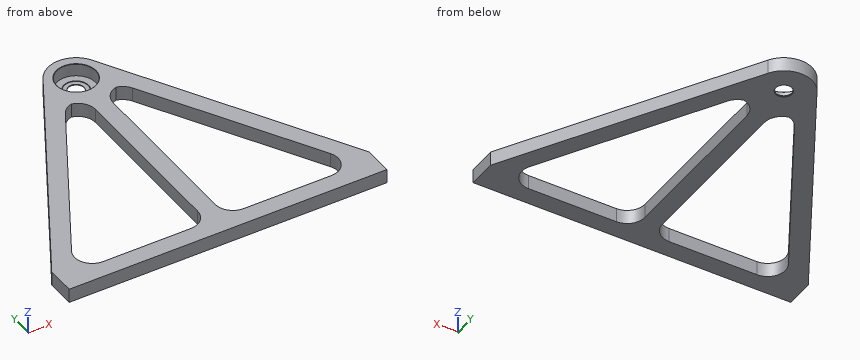
from build123d import *

# Parameters (mm, degrees)
BOSS_EXTRUDE1_DEPTH = 4
SKETCH2_R           = 11.05
CUT_EXTRUDE1_DEPTH  = 7.2
SKETCH3_R           = 7
CUT_EXTRUDE2_DEPTH  = 0.2
SKETCH4_R           = 4.5
CUT_EXTRUDE3_DEPTH  = 186.073210739
CHAMFER1_SIZE       = 0.2
CUT_EXTRUDE4_DEPTH  = 186.09817215
SKETCH8_W           = 10
SKETCH8_H           = 114
EXTRUDE_THIN1_DEPTH = 8
FILLET1_R           = 10
SKETCH6_OUTSIDE_W   = 251.144
SKETCH6_OUTSIDE_H   = 208.536
SKETCH6_OUTSIDE_W_2 = 180
SKETCH6_OUTSIDE_H_2 = 156
CUT_EXTRUDE5_DEPTH  = 186.09817215


# Some blends are built 0.0001 mm under size
with BuildPart() as part:
    # Sketch1 → Boss-Extrude1 (new, symmetric)
    with BuildSketch(Plane.XY):
        with BuildLine():
            Line((0, 0), (-99.304246301, 0))
            Line((-99.304246301, 0), (-13.856406461, 148))
            ThreePointArc((-13.856406461, 148), (0, 156), (13.856406461, 148))
            Line((13.856406461, 148), (99.304246301, 0))
            Line((99.304246301, 0), (0, 0))
        make_face()
    extrude(amount=BOSS_EXTRUDE1_DEPTH, both=True)

    # Sketch2 → Cut-Extrude1 (cut)
    with BuildSketch(Plane.XY.offset(4)):
        with Locations((0, 140)):
            Circle(SKETCH2_R)
    extrude(amount=-CUT_EXTRUDE1_DEPTH, mode=Mode.SUBTRACT)

    # Sketch3 → Cut-Extrude2 (cut)
    with BuildSketch(Plane.XY.offset(-3.2)):
        with Locations((0, 140)):
            Circle(SKETCH3_R)
    extrude(amount=-CUT_EXTRUDE2_DEPTH, mode=Mode.SUBTRACT)

    # Sketch4 → Cut-Extrude3 (cut, through all)
    with BuildSketch(Plane.XY.offset(-3.4)):
        with Locations((0, 140)):
            Circle(SKETCH4_R)
    extrude(amount=-CUT_EXTRUDE3_DEPTH, mode=Mode.SUBTRACT)

    # Chamfer1
    chamfer1_edges = [part.edges().sort_by_distance(p)[0] for p in [
        (-11.05, 140, 4),
        (-7, 140, -3.4),
        (-4.5, 140, -4),
    ]]
    chamfer(chamfer1_edges, length=CHAMFER1_SIZE - 0.0001)  # a hair under: the kernel refuses the full size

    # Sketch5 → Cut-Extrude4 (cut, through all)
    with BuildSketch(Plane.XY.offset(4)):
        Polygon((-16.165807537, 124), (16.165807537, 124), (81.983738225, 10), (-81.983738225, 10), align=None)
    extrude(amount=-CUT_EXTRUDE4_DEPTH, mode=Mode.SUBTRACT)

    # Sketch8 → Extrude-Thin1 (add)
    with BuildSketch(Plane.XY.offset(4)):
        with Locations((0, 67)):
            Rectangle(SKETCH8_W, SKETCH8_H)
    extrude(amount=-EXTRUDE_THIN1_DEPTH)

    # Fillet1
    # the kernel refuses this fillet: 10 mm, written as the material it adds along each edge
    with BuildSketch(Plane(origin=(81.983738225, 10, 4), x_dir=(-0.5000000000000037, 0.8660254037844365, 0), z_dir=(0, 0, -1)), Plane(origin=(-81.983738225, 10, 4), x_dir=(1, 0, 0), z_dir=(0, 0, -1))) as fillet1_piece_1:
        with BuildLine():
            CenterArc((FILLET1_R * 1.73205080757, -FILLET1_R), FILLET1_R, 90, 120)
            Line((FILLET1_R * 0.866025403784, -FILLET1_R * 1.5), (0, 0))
            Line((0, 0), (FILLET1_R * 1.73205080757, 0))
        make_face()
    extrude(amount=8)
    with BuildSketch(Plane(origin=(16.165807537, 124, 4), x_dir=(-1, 0, 0), z_dir=(0, 0, -1))) as fillet1_piece_2:
        with BuildLine():
            CenterArc((FILLET1_R * 0.57735026919, -FILLET1_R), FILLET1_R, 90, 60)
            Line((-FILLET1_R * 0.288675134595, -FILLET1_R * 0.5), (0, 0))
            Line((0, 0), (FILLET1_R * 0.57735026919, 0))
        make_face()
    extrude(amount=8)
    with BuildSketch(Plane(origin=(-16.165807537, 124, 4), x_dir=(1, 0, 0), z_dir=(0, 0, -1))) as fillet1_piece_3:
        with BuildLine():
            CenterArc((FILLET1_R * 0.57735026919, FILLET1_R), FILLET1_R, 210, 60)
            Line((-FILLET1_R * 0.288675134595, FILLET1_R * 0.5), (0, 0))
            Line((0, 0), (FILLET1_R * 0.57735026919, 0))
        make_face()
    extrude(amount=8)
    with BuildSketch(Plane(origin=(-5, 10, 4), x_dir=(-1, 0, 0), z_dir=(0, 0, -1)), Plane(origin=(5, 124, 4), x_dir=(1, 0, 0), z_dir=(0, 0, -1))) as fillet1_piece_4:
        with BuildLine():
            CenterArc((FILLET1_R, FILLET1_R), FILLET1_R, 180, 90)
            Line((0, FILLET1_R), (0, 0))
            Line((0, 0), (FILLET1_R, 0))
        make_face()
    extrude(amount=8)
    with BuildSketch(Plane(origin=(5, 10, 4), x_dir=(1, 0, 0), z_dir=(0, 0, -1)), Plane(origin=(-5, 124, 4), x_dir=(-1, 0, 0), z_dir=(0, 0, -1))) as fillet1_piece_5:
        with BuildLine():
            CenterArc((FILLET1_R, -FILLET1_R), FILLET1_R, 90, 90)
            Line((0, -FILLET1_R), (0, 0))
            Line((0, 0), (FILLET1_R, 0))
        make_face()
    extrude(amount=8)

    # Sketch6 outside → Cut-Extrude5 (cut, through all)
    with BuildSketch(Plane.XY.offset(4)):
        with Locations((0, 78)):
            Rectangle(SKETCH6_OUTSIDE_W, SKETCH6_OUTSIDE_H)
        with Locations((0, 78)):
            Rectangle(SKETCH6_OUTSIDE_W_2, SKETCH6_OUTSIDE_H_2, mode=Mode.SUBTRACT)
    extrude(amount=-CUT_EXTRUDE5_DEPTH, mode=Mode.SUBTRACT)


solid = part.part
Model file for the job. Use its own axes, mm. Coordinates: 2 decimals unless noted, no trailing zeros. Write each loop counter-clockwise with the first axis right and the second up, starting at its lowest first coordinate (ties: lowest second). Pieces come first, ordered by that corner, then holes. Notation, with made-up numbers: (18, -23) -> (40, -23) arc R21 cw to (40, -18) -> close; hole circle Ø9 at (42.25, -5). An arc over 180 degrees is marked (long way). One line per item, written item: value. Start each with the question number.
1) Slice it at A-A on z = -0.25. Write the cut outline in (x, y), then the cut area to 3 significant figures.
2) Slice it at C-C on y = 79. Write the cut outline in (x, z).
3) Probe probe 1 along Y at (x, z) = (0, -0.5); probe 2 along X at (y, z) = (116, -3.5); probe 3 along X at (y, z) = (45, -2.5). List the from-to ranges inside material, lowest first.
4) Flat gauge pins, fed straight in: pin 1 Ø4 at (y, z) = (60, 0.5) entering from -X; pin 2 Ø4 at (x, z) = (47.5, -2) entering from -Y; pin 3 Ø4 at (x, z) = (38, -1.5) entering from +Y; pin 4 Ø13.5 at (x, y) = (0, 140) entering from +Z. Where does each tip first touch, or does it go through?
Answers follow:
1. outline: (-90, 0) -> (90, 0) -> (90, 16.12) -> (13.86, 148) arc R16 ccw to (-13.86, 148) -> (-90, 16.12) -> close; hole (-73.32, 25) arc R10 ccw to (-64.66, 10) -> (-15, 10) arc R10 ccw to (-5, 20) -> (-5, 114) arc R10 ccw to (-12.7, 123.73) arc R10 ccw to (-19.05, 119) -> close; hole circle Ø22.1 at (0, 140); hole (5, 20) arc R10 ccw to (15, 10) -> (64.66, 10) arc R10 ccw to (73.32, 25) -> (19.05, 119) arc R10 ccw to (12.7, 123.73) arc R10 ccw to (5, 114) -> close
1. area: 6,560 mm2
2. outline: (-53.69, -4) -> (-42.15, -4) -> (-42.15, 4) -> (-53.69, 4) -> close; (-5, -4) -> (5, -4) -> (5, 4) -> (-5, 4) -> close; (42.15, -4) -> (53.69, -4) -> (53.69, 4) -> (42.15, 4) -> close
3. probe 1: 0 to 128.95, 151.05 to 156
3. probe 2: -32.33 to -20.78, -5.2 to 5.2, 20.78 to 32.33
3. probe 3: -73.32 to -61.78, -5 to 5, 61.78 to 73.32
4. pin 1: x = -65.82
4. pin 2: y = 0
4. pin 3: y = 109.65
4. pin 4: z = -3.4
